The model under review builds one solid part; all positions refer to its coordinate system, in mm. Face numbers are marked on the shaded views. A direction names the side the tool comes from. Round coordinates to 2 decimals unless told otherwise and drop trailing zeros. Loops run counter-clockwise (first coordinate to the right, second up) from the corner with the lowest first, then second, coordinate; pieces in that order, holes last. Notation, with made-up numbers: (59.25, 43.25) - (116.25, 43.25) arc R31 cw to (116.25, 81.25) - close; hole circle Ø1 at (40.25, -16). An arc over 180 degrees is marked (long way). Answer as CSV lines item,"result".
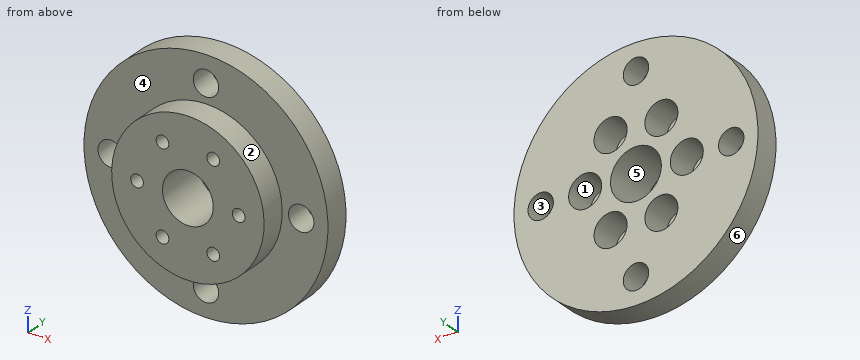
from build123d import *

# Parameters (mm, degrees)
SKETCH1_R           = 15
BOSS_EXTRUDE1_DEPTH = 5
SKETCH3_R           = 24
BOSS_EXTRUDE3_DEPTH = 5
SKETCH2_R           = 1.25
SKETCH2_R_2         = 5
CUT_EXTRUDE1_DEPTH  = 11.5
SKETCH4_R           = 3.25
CUT_EXTRUDE2_DEPTH  = 6
SKETCH5_R           = 2.5
CUT_EXTRUDE3_DEPTH  = 6.5


with BuildPart() as part:
    # Sketch1 → Boss-Extrude1 (new body)
    with BuildSketch(Plane(origin=(0, 0, 0), x_dir=(1, 0, 0), z_dir=(0, 1, 0))):
        with Locations(Location((0, 0, 0), (0, 0, 270))):
            Circle(SKETCH1_R)
    extrude(amount=BOSS_EXTRUDE1_DEPTH)

    # Sketch3 → Boss-Extrude3 (add)
    with BuildSketch(Plane(origin=(0, 5, 0), x_dir=(1, 0, 0), z_dir=(0, 1, 0))):
        with Locations(Location((0, 0, 0), (0, 0, 270))):
            Circle(SKETCH3_R)
    extrude(amount=BOSS_EXTRUDE3_DEPTH)

    # Sketch2 → Cut-Extrude1 (cut)
    with BuildSketch(Plane(origin=(0, 0, 0), x_dir=(1, 0, 0), z_dir=(0, 1, 0))):
        with Locations(Location((-5, 8.660254038, 0), (0, 0, 270))):
            Circle(SKETCH2_R)
        with Locations(Location((5, 8.660254038, 0), (0, 0, 270))):
            Circle(SKETCH2_R)
        with Locations(Location((10, 0, 0), (0, 0, 270))):
            Circle(SKETCH2_R)
        with Locations(Location((5, -8.660254038, 0), (0, 0, 270))):
            Circle(SKETCH2_R)
        with Locations(Location((-5, -8.660254038, 0), (0, 0, 270))):
            Circle(SKETCH2_R)
        with Locations(Location((-10, 0, 0), (0, 0, 270))):
            Circle(SKETCH2_R)
        with Locations(Location((0, 0, 0), (0, 0, 270))):
            Circle(SKETCH2_R_2)
    extrude(amount=CUT_EXTRUDE1_DEPTH, mode=Mode.SUBTRACT)

    # Sketch4 → Cut-Extrude2 (cut)
    with BuildSketch(Plane(origin=(0, 10, 0), x_dir=(1, 0, 0), z_dir=(0, 1, 0))):
        with Locations(Location((10, 0, 0), (0, 0, 270))):
            Circle(SKETCH4_R)
        with Locations(Location((5, 8.660254038, 0), (0, 0, 270))):
            Circle(SKETCH4_R)
        with Locations(Location((5, -8.660254038, 0), (0, 0, 270))):
            Circle(SKETCH4_R)
        with Locations(Location((-5, -8.660254038, 0), (0, 0, 270))):
            Circle(SKETCH4_R)
        with Locations(Location((-10, 0, 0), (0, 0, 270))):
            Circle(SKETCH4_R)
        with Locations(Location((-5, 8.660254038, 0), (0, 0, 270))):
            Circle(SKETCH4_R)
    extrude(amount=-CUT_EXTRUDE2_DEPTH, mode=Mode.SUBTRACT)

    # Sketch5 → Cut-Extrude3 (cut)
    with BuildSketch(Plane(origin=(0, 10, 0), x_dir=(1, 0, 0), z_dir=(0, 1, 0))):
        with Locations(Location((0, 18.75, 0), (0, 0, 270))):
            Circle(SKETCH5_R)
        with Locations(Location((18.75, 0, 0), (0, 0, 270))):
            Circle(SKETCH5_R)
        with Locations(Location((0, -18.75, 0), (0, 0, 270))):
            Circle(SKETCH5_R)
        with Locations(Location((-18.75, 0, 0), (0, 0, 270))):
            Circle(SKETCH5_R)
    extrude(amount=-CUT_EXTRUDE3_DEPTH, mode=Mode.SUBTRACT)


solid = part.part
1. Take a section at B-B (y = 2). State the section outline as (x, z) points, plus the area to 3 significant figures.
Numbers:
outline,"circle Ø30 at (0, 0); hole circle Ø2.5 at (-10, 0); hole circle Ø2.5 at (-5, -8.66); hole circle Ø2.5 at (-5, 8.66); hole circle Ø10 at (0, 0); hole circle Ø2.5 at (5, -8.66); hole circle Ø2.5 at (5, 8.66); hole circle Ø2.5 at (10, 0)"
area,"599 mm²"
2. Tool access review of the marked faces 1, 2 and 3: name each direction out of +Z, -Z, +X, -X, +Y, -Y from which nothing blocks a thin tool from reaching the whole face with its end or side.
Numbers:
face 1,"+Y"
face 2,"-Y"
face 3,"+Y, -Y"
3. Take a section at A-A (x = 0). State the section outline as (y, z) points.
Numbers:
outline,"(0, -15) - (5, -15) - (5, -16.25) - (10, -16.25) - (10, -5) - (0, -5) - close; (0, 5) - (10, 5) - (10, 16.25) - (5, 16.25) - (5, 15) - (0, 15) - close; (5, -24) - (10, -24) - (10, -21.25) - (5, -21.25) - close; (5, 21.25) - (10, 21.25) - (10, 24) - (5, 24) - close"
4. Draft analysis for pull direction Z (two halves, no side actions). For the marked faces 4, 5 and 6, state which applies: +Z half, -Z half, draft (parallel to the pull), parting line (faces both ways), or undercut.
Numbers:
face 4,"draft"
face 5,"undercut"
face 6,"parting line"
5. Take a section at D-D (z = 18.75). State the section outline as (x, y) points.
Numbers:
outline,"(-14.98, 5) - (-2.5, 5) - (-2.5, 10) - (-14.98, 10) - close; (2.5, 5) - (14.98, 5) - (14.98, 10) - (2.5, 10) - close"
6. Wall thickness on probe 1 along X at (y, z) = (8.45, 0); probe 2 along X at (y, z) = (2.6, 0); probe 3 along X at (y, z) = (7.5, -8): over which ranges is each line inside the solid? List them lowest first.
Numbers:
probe 1,"x = -24 to -21.25, -16.25 to -13.25, -6.75 to -5, 5 to 6.75, 13.25 to 16.25, 21.25 to 24"
probe 2,"x = -15 to -11.25, -8.75 to -5, 5 to 8.75, 11.25 to 15"
probe 3,"x = -22.63 to -8.18, -1.82 to 1.82, 8.18 to 22.63"
7. Clearance check with flat-ended pins moving along their axes: pin 1 (2 mm diameter, centred on x = -10, z = 0, fed in from +Y); pin 2 (1 mm diameter, centred on x = 12, y = 8.5, fed in from -Z); pin 3 (3 mm diameter, centred on x = -6.5, y = 4, fed in from -Z); pin 4 (5 mm diameter, centred on y = 7.5, z = -10, fed in from +X). State where each tip first meets the part, or that it passes through.
Numbers:
pin 1,"passes through"
pin 2,"stops at z = -21.07"
pin 3,"stops at z = -23.39"
pin 4,"stops at x = 22.8"
8. Take a section at C-C (y = 7.5). State how many separate pieces and enclosed holes the cut face has, plus the area to 3 significant figures.
Numbers:
separate pieces,"1"
enclosed holes,"11"
area,"1,450 mm²"
